Verification items for the finished model (mm, model axes). A direction names the side the tool comes from. Round coordinates to 2 decimals unless told otherwise and drop trailing zeros. Order: outer loops, then holes, each group sorted by start corner. A loop starts at its lowest first (then second) coordinate and runs counter-clockwise, first axis right, second up. Notation, with made-up numbers: (45.25, -21) -> (98.25, -21) arc R24 cw to (98.25, -4) -> close; hole circle Ø4 at (52, 84). An arc over 180 degrees is marked (long way). Answer in a Markdown table with one row per item. Add a question column.
Autodesk Inventor part; units mm, degrees
ref_plane "YZ Plane" through (0, 0, 0) normal (1, 0, 0) x (0, 1, 0)
ref_plane "XZ Plane" through (0, 0, 0) normal (0, 1, 0) x (-1, 0, 0)
ref_plane "XY Plane" through (0, 0, 0) normal (0, 0, 1) x (1, 0, 0)
sketch "Sketch1" plane through (0, 0, 0) normal (0, 1, 0) x (-1, 0, 0)
  line L0 (-9, 20) -> (9, 20)
  line L1 (9, 20) -> (9, -20)
  line L2 (9, -20) -> (-9, -20)
  line L3 (-9, -20) -> (-9, 20)
  line L4 (-9, 20) -> (9, -20) construction
  line L5 (9, 20) -> (-9, -20) construction
  point P0 (0, 0)
  dimension "d0" = 18
  dimension "d1" = 40
extrude "Extrusion1" add sketch "Sketch1" along normal blind 7
sketch "Sketch2" plane through (0, 7, 0) normal (0, 1, 0) x (1, 0, 0)
  circle A0 centre (1, -12.5) radius 3.1
  line L0 (-9, -20) -> (9, -20)
  line L1 (9, -20) -> (9, 20)
  point P0 (0, 0)
  dimension "d4" = 6.2
  dimension "d5" = 7.5
  dimension "d6" = 8
extrude "Extrusion2" cut sketch "Sketch2" against normal through all
mirror "Mirror1" about plane through (0, 0, 0) normal (0, 0, 1) of "Extrusion2"
sketch "Sketch3" plane through (9, 0, 20) normal (1, 0, 0) x (0, 0, -1)
  line L0 (0, 7) -> (40, 7)
  line L1 (16, 7) -> (12.4645, 3.4645)
  line L2 (16, 7) -> (21, 7) construction
  line L3 (16, 7) -> (24, 7)
  line L4 (16, 7) -> (24, 7) construction
  line L5 (24, 7) -> (27.5355, 3.4645)
  line L6 (27.5355, 3.4645) -> (12.4645, 3.4645)
  point P0 (20, 0)
  dimension "d9" = 5
  dimension "d10" = 135
  dimension "d11" = 16
  dimension "d12" = 8
  dimension "d13" = 0
  dimension "d14" = 5
  dimension "d15" = 135
extrude "Extrusion3" cut sketch "Sketch3" against normal blind 10
fillet "Fillet1" radius 1 3 edges at (0, 7, -20) (-9, 7, 0) (0, 7, 20)
properties part number "Dovetail_holder_V2"
1) Cross-section at B-B, the plane y = 4.5. Record the boundary of the cut face in (x, z).
2) Thickness scan on L1, parallel to Z at x = 1, y = 3.25; L2, parallel to X at y = 2.25, z = 12.5; L3, parallel to Y at x = -0.5, z = -5. Record the ranges inside material, lowest first. Write a range as [from, to].
3) Tool access check on faces 1 (the face through (4, 5, 6)), 2 (the face through (-8.715, 6.699, -0.28)). Record the directions out of +Z, -Z, +X, -X, +Y, -Y that give a thin tool (end or side, any length) a straight path to the whole face; none if there is none.
4) Cross-section at C-C, the plane x = 1. Record the boundary of the cut face in (y, z), and give its area (3 significant figures).
5) Draft check along X on faces 3 (the face through (2.43, 3.55, 15.25)), 4 (the face through (-9, 3, 0)), 5 (the face through (4, 5, -6)). Enter one of: +X half, -X half, draft (parallel to the pull), parting line (faces both ways), or undercut.
6) Depth check by flat-ended pin: P1, Ø3, axis at x = 2, z = 0, coming from the +Y side; P2, Ø1.1, axis at y = 4.5, z = 3.5, coming from the +X side. Enter the tip coordinate at first touch or a pass-through.
7) Cross-section at D-D, the plane z = 0. Record the boundary of the cut face in (x, y).
8) Cross-section at A-A, the plane z = -12.5. Record the boundary of the cut face in (x, y), and give its area (3 significant figures).
Results below:
| question | item | result |
|---|---|---|
| 1 | outline | (-9, -20) -> (9, -20) -> (9, -6.5) -> (-1, -6.5) -> (-1, 6.5) -> (9, 6.5) -> (9, 20) -> (-9, 20) -> close; hole circle Ø6.2 at (1, -12.5); hole circle Ø6.2 at (1, 12.5) |
| 2 | L1 | [-20, -15.6], [-9.4, 9.4], [15.6, 20] |
| 2 | L2 | [-9, -2.1], [4.1, 9] |
| 2 | L3 | [0, 3.46], [6, 7] |
| 3 | face 1 | +X |
| 3 | face 2 | +Z, -Z, -X, +Y |
| 4 | outline | (0, -20) -> (6, -20) arc R1 ccw to (7, -19) -> (7, -15.6) -> (0, -15.6) -> close; (0, -9.4) -> (7, -9.4) -> (7, -4) -> (3.46, -7.54) -> (3.46, 7.54) -> (7, 4) -> (7, 9.4) -> (0, 9.4) -> close; (0, 15.6) -> (7, 15.6) -> (7, 19) arc R1 ccw to (6, 20) -> (0, 20) -> close |
| 4 | area | 152 mm² |
| 5 | face 3 | undercut |
| 5 | face 4 | -X half |
| 5 | face 5 | draft |
| 6 | P1 | y = 3.46 |
| 6 | P2 | x = -1 |
| 7 | outline | (-9, 0) -> (9, 0) -> (9, 3.46) -> (-1, 3.46) -> (-1, 7) -> (-8, 7) arc R1 ccw to (-9, 6) -> close |
| 8 | outline | (-9, 0) -> (-2.1, 0) -> (-2.1, 7) -> (-8, 7) arc R1 ccw to (-9, 6) -> close; (4.1, 0) -> (9, 0) -> (9, 7) -> (4.1, 7) -> close |
| 8 | area | 82.4 mm² |
